```python
from build123d import *

# Parameters (mm, degrees)
SKETCH1_R                            = 4.7625
BOSS_EXTRUDE1_DEPTH                  = 60.325
F_10_32_TAPPED_HOLE1_D               = 4.0386
F_10_32_TAPPED_HOLE1_DEPTH           = 16.256
F_10_32_TAPPED_HOLE1_TIP             = 1.213317848
F_10_32_TAPPED_HOLE1_ON_FACE_2_D     = 4.0386
F_10_32_TAPPED_HOLE1_ON_FACE_2_DEPTH = 16.256
F_10_32_TAPPED_HOLE1_ON_FACE_2_TIP   = 1.213317848


with BuildPart() as part:
    # Sketch1 → Boss-Extrude1 (new, symmetric)
    with BuildSketch(Plane(origin=(0, 0, 0), x_dir=(0, 0, -1), z_dir=(1, 0, 0))):
        with Locations(Location((0, 0, 0), (0, 0, 180))):
            Circle(SKETCH1_R)
    extrude(amount=BOSS_EXTRUDE1_DEPTH, both=True)

    # #10-32 Tapped Hole1
    with Locations(Plane(origin=(60.325, 0, 0), x_dir=(0, 0, 1), z_dir=(1, 0, 0))):
        with Locations((0, 0)):
            Hole(F_10_32_TAPPED_HOLE1_D / 2, depth=F_10_32_TAPPED_HOLE1_DEPTH)
            with Locations((0, 0, -(F_10_32_TAPPED_HOLE1_DEPTH + F_10_32_TAPPED_HOLE1_TIP / 2))):  # 118° drill point
                Cone(0, F_10_32_TAPPED_HOLE1_D / 2, F_10_32_TAPPED_HOLE1_TIP, mode=Mode.SUBTRACT)

    # #10-32 Tapped Hole1 on face 2
    with Locations(Plane(origin=(-60.325, 0, 0), x_dir=(0, 0, -1), z_dir=(-1, 0, 0))):
        with Locations((0, 0)):
            Hole(F_10_32_TAPPED_HOLE1_ON_FACE_2_D / 2, depth=F_10_32_TAPPED_HOLE1_ON_FACE_2_DEPTH)
            with Locations((0, 0, -(F_10_32_TAPPED_HOLE1_ON_FACE_2_DEPTH + F_10_32_TAPPED_HOLE1_ON_FACE_2_TIP / 2))):  # 118° drill point
                Cone(0, F_10_32_TAPPED_HOLE1_ON_FACE_2_D / 2, F_10_32_TAPPED_HOLE1_ON_FACE_2_TIP, mode=Mode.SUBTRACT)


solid = part.part
```
Here's how the part is built. I have some questions about the finished solid (model axes, mm). A direction names the side the tool comes from. Round coordinates to 2 decimals unless told otherwise and drop trailing zeros. Loops run counter-clockwise (first coordinate to the right, second up) from the corner with the lowest first, then second, coordinate; pieces in that order, holes last. Notation, with made-up numbers: (-12, 5.5) -> (19, 5.5) arc R32 ccw to (19, 42.5) -> close; hole circle Ø5 at (-22, 84). An arc over 180 degrees is marked (long way). Answer as CSV lines item,"result". Start each with the question number.
1. I'm going to push flat-ended pins straight in: P1, Ø5, axis at x = -38, z = -3.5, coming from the +Y side; P2, Ø3, axis at x = 6.5, z = 3, coming from the +Y side; P3, Ø3.5, axis at y = 0, z = 0, coming from the +X side. Where does each tip first touch, or does it pass through?
2. Imagine slicing it at B-B on x = -29. Write out the boundary of the cut face in (y, z) (1 decimal).
3. If we mould it in two halves opening along Z, with no side actions, what happens to faces 3 (the face through (52.083, -0.607, -1.926)), 4 (the face through (0.84, 4.65, -1.03)), 5 (the face through (60.325, 1, 2))? For each: pulls with the +Z half, pulls with the -Z half, needs draft (parallel to the pull), parting line crosses it, or undercut.
4. Imagine slicing it at C-C on y = -3.5. Write out the boundary of the cut face in (x, z) (3 decimals), plus the area to 3 significant figures.
5. Imagine slicing it at A-A on z = -3.25. Write out the boundary of the cut face in (x, y) (3 decimals).
6. I need wall thicknesses on probe 1 along Y at (x, z) = (-48.25, 0); probe 2 along Y at (x, z) = (5, -3.25); probe 3 along Y at (x, z) = (24.5, -2.25). Which ranges of each line are inside material? Lowest first, please. Write a range as from..to.
7. For faces 1 (the face through (-60.325, 1, 2)), 2 (the face through (-52.083, -0.607, 1.926)), which set-ups out of +Z, -Z, +X, -X, +Y, -Y let a thin tool reach every point of the face, with its end or its side?
Solution:
1,P1,"y = 4.66"
1,P2,"y = 4.52"
1,P3,"x = 43.91"
2,outline,"circle Ø9.5 at (0, 0)"
3,face 3,"undercut"
3,face 4,"parting line crosses it"
3,face 5,"needs draft"
4,outline,"(-60.325, -3.23) -> (60.325, -3.23) -> (60.325, 3.23) -> (-60.325, 3.23) -> close"
4,area,"779 mm²"
5,outline,"(-60.325, -3.481) -> (60.325, -3.481) -> (60.325, 3.481) -> (-60.325, 3.481) -> close"
6,probe 1,"-4.76..-2.02, 2.02..4.76"
6,probe 2,"-3.48..3.48"
6,probe 3,"-4.2..4.2"
7,face 1,"+Z, -Z, -X, +Y, -Y"
7,face 2,"-X"
